Work out the finished part from the listing and answer in its coordinate system (mm). A direction names the side the tool comes from. Coordinates: 2 decimals unless noted, no trailing zeros. Loops run counter-clockwise (first coordinate to the right, second up) from the corner with the lowest first, then second, coordinate; pieces in that order, holes last. Notation, with made-up numbers: (60, -24) -> (69, -24) arc R16 cw to (69, -6) -> close; hole circle Ø5 at (5.25, 61.25). An arc over 180 degrees is marked (long way). One line per question, with ' | ' between items.
```python
from build123d import *

# Parameters (mm, degrees)
F1_DEPTH = 12.7


with BuildPart() as f1:
    # F0 (on Top) → F1 (new body)
    with BuildSketch(Plane.XY):
        Polygon((12.7, -12.7), (25.4, -12.7), (25.4, 0), (38.1, 0), (38.1, 12.7), (50.8, 12.7), (50.8, 25.4), (63.5, 25.4), (63.5, 38.1), (76.2, 38.1), (76.2, 50.8), (88.9, 50.8), (88.9, 63.5), (101.6, 63.5), (101.6, 101.6), (88.9, 101.6), (76.2, 101.6), (63.5, 101.6), (63.5, 88.9), (50.8, 88.9), (50.8, 76.2), (38.1, 76.2), (38.1, 63.5), (25.4, 63.5), (25.4, 50.8), (12.7, 50.8), (12.7, 38.1), (0, 38.1), (0, 25.4), (-12.7, 25.4), (-12.7, 12.7), (-25.4, 12.7), (-25.4, 0), (-38.1, 0), (-38.1, 12.7), (-50.8, 12.7), (-50.8, 25.4), (-76.2, 25.4), (-76.2, 0), (-63.5, 0), (-63.5, -25.4), (-50.8, -25.4), (-50.8, -38.1), (-63.5, -38.1), (-63.5, -50.8), (-76.2, -50.8), (-76.2, -63.5), (-101.6, -63.5), (-101.6, -76.2), (-101.6, -88.9), (-101.6, -101.6), (-63.5, -101.6), (-63.5, -76.2), (-50.8, -76.2), (-50.8, -63.5), (-38.1, -63.5), (-38.1, -50.8), (-25.4, -50.8), (-25.4, -63.5), (0, -63.5), (0, -76.2), (25.4, -76.2), (25.4, -63.5), (25.4, -50.8), (12.7, -50.8), (12.7, -38.1), (0, -38.1), (0, -25.4), (12.7, -25.4), align=None)
    extrude(amount=F1_DEPTH)


solid = f1.part
```
1) For faces 1 (the face through (0, 32, 6)), 2 (the face through (-70, 0, 6)), 3 (the face through (6, -38.1, 6)), 4 (the face through (57, 25.4, 6)), determine the directions among +Z, -Z, +X, -X, +Y, -Y from which every point of the face is accessible in a straight line to the end or side of a thin tool.
Check values:
face 1: +Z, -Z, -X, +Y | face 2: +Z, -Z, -X | face 3: +Z, -Z, +X | face 4: +Z, -Z, +X, -Y
2) Find section D-D (y = 68). Write down the section's boundary in (x, z), plus the area to 3 significant figures.
Check values:
outline: (38.1, 0) -> (101.6, 0) -> (101.6, 12.7) -> (38.1, 12.7) -> close | area: 806 mm^2
3) The mould has two halves that part along Y. Classify faces 5 (the face through (95, 63.5, 6)), 6 (the face through (-63.5, -13, 6)), 7 (the face through (25.4, -6, 6)): released by +Y, released by -Y, zero draft, split by the parting line, or undercut.
Check values:
face 5: released by -Y | face 6: undercut | face 7: zero draft
4) Find section C-C (x = -34.5). Write down the section's boundary in (y, z).
Check values:
outline: (-50.8, 0) -> (0, 0) -> (0, 12.7) -> (-50.8, 12.7) -> close
5) Find the intervals of material crossed by line 1 along Y through (x, z) = (-52, 3); line 2 along X through (y, z) = (-64.5, 9); line 3 along Y through (x, z) = (16, 7.5), in increasing order.
Check values:
line 1: y = -76.2 to -38.1, -25.4 to 25.4 | line 2: x = -101.6 to -50.8, 0 to 25.4 | line 3: y = -76.2 to -50.8, -12.7 to 50.8
6) Flat-ended cylindrical pins translate along their axes: pin 1 (5 mm diameter, centred on x = -29, z = 11.5, fed in from -Y); pin 2 (6.5 mm diameter, centred on x = -94, z = 6.5, fed in from +Y); pin 3 (6.5 mm diameter, centred on y = 22, z = 7.5, fed in from -X). Find the tip coordinate at first contact, or state that the pin passes through.
Check values:
pin 1: stops at y = -50.8 | pin 2: stops at y = -63.5 | pin 3: stops at x = -76.2
7) Find section A-A (y = -56). Write down the section's boundary in (x, z).
Check values:
outline: (-76.2, 0) -> (-38.1, 0) -> (-38.1, 12.7) -> (-76.2, 12.7) -> close; (-25.4, 0) -> (25.4, 0) -> (25.4, 12.7) -> (-25.4, 12.7) -> close
